from build123d import *

# Parameters (mm, degrees)
SKETCH1_W           = 65
SKETCH1_H           = 32
BOSS_EXTRUDE1_DEPTH = 12
SKETCH10_R          = 3.25
BOLT_EXTRUDE_DEPTH  = 12
SKETCH7_W           = 58
SKETCH7_H           = 27
CUT_EXTRUDE5_DEPTH  = 8
SKETCH8_W           = 5
SKETCH8_H           = 32
BOSS_EXTRUDE3_DEPTH = 11
FILLET6_START       = 3
FILLET6_DEPTH       = 9
FILLET6_START_2     = -16
FILLET6_2_DEPTH     = 4
FILLET6_START_3     = 15
FILLET6_3_DEPTH     = 1
FILLET6_4_ANGLE     = 90
FILLET6_5_ANGLE     = 90
FILLET6_6_ANGLE     = 90
FILLET6_7_ANGLE     = 90
FILLET9_R           = 1
SKETCH11_W          = 120
SKETCH11_H          = 6.033066078
BOSS_EXTRUDE4_DEPTH = 10
SKETCH12_R          = 3.25
BOSS_EXTRUDE5_DEPTH = 12
FILLET11_R          = 7
FILLET12_R          = 3
FILLET13_R          = 3
FILLET15_R          = 1
FILLET16_R          = 1


with BuildPart() as part:
    # Sketch1 → Boss-Extrude1 (new body)
    with BuildSketch(Plane(origin=(0, 0, 0), x_dir=(1, 0, 0), z_dir=(0, 1, 0))):
        with Locations((-32.5, 0)):
            Rectangle(SKETCH1_W, SKETCH1_H)
    extrude(amount=BOSS_EXTRUDE1_DEPTH)

    # Sketch10 → bolt extrude (add)
    with BuildSketch(Plane(origin=(0, 12, 0), x_dir=(1, 0, 0), z_dir=(0, 1, 0))):
        with BuildLine():
            Line((-65, 16), (-70, 16))
            ThreePointArc((-70, 16), (-76.652203093, 14.551570156), (-82.1, 10.468524251))
            Line((-82.1, 10.468524251), (-82.1, -10.468524251))
            ThreePointArc((-82.1, -10.468524251), (-76.652203093, -14.551570156), (-70, -16))
            Line((-70, -16), (-65, -16))
            Line((-65, -16), (-65, 16))
        make_face()
        with Locations(Location((-70.1, -1, 0), (0, 0, 270))):
            Circle(SKETCH10_R, mode=Mode.SUBTRACT)
    extrude(amount=-BOLT_EXTRUDE_DEPTH)

    # Sketch7 → Cut-Extrude5 (cut)
    with BuildSketch(Plane(origin=(0, 12, 0), x_dir=(1, 0, 0), z_dir=(0, 1, 0))):
        with Locations((-29, -1.5)):
            Rectangle(SKETCH7_W, SKETCH7_H)
    extrude(amount=-CUT_EXTRUDE5_DEPTH, mode=Mode.SUBTRACT)

    # Mirror1: part across plane


with BuildPart() as part_1:
    add(part.part)
    add(part.part.mirror(Plane(origin=(0, 0, 0), x_dir=(0, 0, 1), z_dir=(1, 0, 0))))

    # Sketch8 → Boss-Extrude3 (add)
    with BuildSketch(Plane(origin=(0, 4, 0), x_dir=(1, 0, 0), z_dir=(0, 1, 0))):
        Rectangle(SKETCH8_W, SKETCH8_H)
    extrude(amount=BOSS_EXTRUDE3_DEPTH)

    # Fillet6: read off the stored shape, not the designer's step
    # Fillet6 outline → Fillet6 (add)
    with BuildSketch(Plane(origin=(0, 0, 0), x_dir=(1, 0, 0), z_dir=(0, 1, 0)).offset(FILLET6_START)):
        with BuildLine():
            Line((-2.5, -15), (-2.5, -14))
            ThreePointArc((-2.5, -14), (-2.792893219, -14.707106781), (-3.5, -15))
            Line((-3.5, -15), (-2.5, -15))
        make_face()
        with BuildLine():
            ThreePointArc((-3.5, 12), (-2.792893219, 11.707106781), (-2.5, 11))
            Line((-2.5, 11), (-2.5, 12))
            Line((-2.5, 12), (-3.5, 12))
        make_face()
        with BuildLine():
            Line((-58, -15), (-57, -15))
            ThreePointArc((-57, -15), (-57.707106781, -14.707106781), (-58, -14))
            Line((-58, -14), (-58, -15))
        make_face()
        with BuildLine():
            ThreePointArc((-58, 11), (-57.707106781, 11.707106781), (-57, 12))
            Line((-57, 12), (-58, 12))
            Line((-58, 12), (-58, 11))
        make_face()
        with BuildLine():
            Line((2.5, -14), (2.5, -15))
            Line((2.5, -15), (3.5, -15))
            ThreePointArc((3.5, -15), (2.792893219, -14.707106781), (2.5, -14))
        make_face()
        with BuildLine():
            Line((3.5, 12), (2.5, 12))
            Line((2.5, 12), (2.5, 11))
            ThreePointArc((2.5, 11), (2.792893219, 11.707106781), (3.5, 12))
        make_face()
        with BuildLine():
            ThreePointArc((58, -14), (57.707106781, -14.707106781), (57, -15))
            Line((57, -15), (58, -15))
            Line((58, -15), (58, -14))
        make_face()
        with BuildLine():
            Line((58, 12), (57, 12))
            ThreePointArc((57, 12), (57.707106781, 11.707106781), (58, 11))
            Line((58, 11), (58, 12))
        make_face()
    extrude(amount=FILLET6_DEPTH)

    # Fillet6 2 outline → Fillet6 2 (add)
    with BuildSketch(Plane.XY.offset(FILLET6_START_2)):
        with BuildLine():
            Line((-2.5, 12), (-2.5, 13))
            ThreePointArc((-2.5, 13), (-2.792893219, 12.292893219), (-3.5, 12))
            Line((-3.5, 12), (-2.5, 12))
        make_face()
        with BuildLine():
            ThreePointArc((3.5, 12), (2.792893219, 12.292893219), (2.5, 13))
            Line((2.5, 13), (2.5, 12))
            Line((2.5, 12), (3.5, 12))
        make_face()
    extrude(amount=FILLET6_2_DEPTH)

    # Fillet6 3 outline → Fillet6 3 (add)
    with BuildSketch(Plane.XY.offset(FILLET6_START_3)):
        with BuildLine():
            Line((-2.5, 12), (-2.5, 13))
            ThreePointArc((-2.5, 13), (-2.792893219, 12.292893219), (-3.5, 12))
            Line((-3.5, 12), (-2.5, 12))
        make_face()
        with BuildLine():
            ThreePointArc((3.5, 12), (2.792893219, 12.292893219), (2.5, 13))
            Line((2.5, 13), (2.5, 12))
            Line((2.5, 12), (3.5, 12))
        make_face()
    extrude(amount=FILLET6_3_DEPTH)

    # Fillet6 4 outline → Fillet6 4 (revolve)
    with BuildSketch(Plane(origin=(0, 12, 15), x_dir=(0, 0, -1), z_dir=(0, -1, 0))):
        with BuildLine():
            ThreePointArc((0, -3.5), (0.292893219, -2.792893219), (1, -2.5))
            Line((1, -2.5), (0, -2.5))
            Line((0, -2.5), (0, -3.5))
        make_face()
    revolve(axis=Axis((0, 12, 15), (1, 0, 0)), revolution_arc=FILLET6_4_ANGLE)

    # Fillet6 5 outline → Fillet6 5 (revolve)
    with BuildSketch(Plane(origin=(0, 12, -12), x_dir=(0, 1, 0), z_dir=(0, 0, -1))):
        with BuildLine():
            ThreePointArc((0, -3.5), (0.292893219, -2.792893219), (1, -2.5))
            Line((1, -2.5), (0, -2.5))
            Line((0, -2.5), (0, -3.5))
        make_face()
    revolve(axis=Axis((0, 12, -12), (1, 0, 0)), revolution_arc=FILLET6_5_ANGLE)

    # Fillet6 6 outline → Fillet6 6 (revolve)
    with BuildSketch(Plane(origin=(0, 12, -12), x_dir=(0, 1, 0), z_dir=(0, 0, -1))):
        with BuildLine():
            Line((0, 2.5), (1, 2.5))
            ThreePointArc((1, 2.5), (0.292893219, 2.792893219), (0, 3.5))
            Line((0, 3.5), (0, 2.5))
        make_face()
    revolve(axis=Axis((0, 12, -12), (1, 0, 0)), revolution_arc=FILLET6_6_ANGLE)

    # Fillet6 7 outline → Fillet6 7 (revolve)
    with BuildSketch(Plane(origin=(0, 12, 15), x_dir=(0, 0, -1), z_dir=(0, -1, 0))):
        with BuildLine():
            Line((0, 2.5), (1, 2.5))
            ThreePointArc((1, 2.5), (0.292893219, 2.792893219), (0, 3.5))
            Line((0, 3.5), (0, 2.5))
        make_face()
    revolve(axis=Axis((0, 12, 15), (1, 0, 0)), revolution_arc=FILLET6_7_ANGLE)

    # Fillet9
    fillet9_edges = [part_1.edges().sort_by_distance(p)[0] for p in [
        (2.5, 15, 0),
        (0, 15, -16),
        (-2.5, 15, 0),
        (0, 15, 16),
    ]]
    fillet(fillet9_edges, radius=FILLET9_R)

    # Sketch11 → Boss-Extrude4 (add)
    with BuildSketch(Plane.XZ):
        Polygon((70.002161454, 12.077158354), (-70.005398194, 12), (-70, 16), (70, 16), align=None)
        Rectangle(SKETCH11_W, SKETCH11_H)
        Polygon((70.002161454, -12.077158354), (70, -16), (-70, -16), (-70.005398194, -12), align=None)
    extrude(amount=BOSS_EXTRUDE4_DEPTH)

    # Sketch12 → Boss-Extrude5 (add)
    with BuildSketch(Plane.XZ):
        with BuildLine():
            Line((-8, -12), (-8, -22))
            ThreePointArc((-8, -22), (0, -30), (8, -22))
            Line((8, -22), (8, -12))
            Line((8, -12), (-8, -12))
        make_face()
        with Locations(Location((0, -22, 0), (0, 0, 270))):
            Circle(SKETCH12_R, mode=Mode.SUBTRACT)
    extrude(amount=-BOSS_EXTRUDE5_DEPTH)

    # Fillet11
    fillet11_edges = [part_1.edges().sort_by_distance(p)[0] for p in [
        (-70.002699097, 0, -14),
        (70.001080727, 0, -14.038579177),
        (-70.002699097, 0, 14),
        (70.001080727, 0, 14.038579177),
    ]]
    fillet(fillet11_edges, radius=FILLET11_R)

    # Fillet12
    fillet12_edges = [part_1.edges().sort_by_distance(p)[0] for p in [
        (0, 0, 3.016533039),
        (0, 0, -3.016533039),
        (-0.001624692, 0, 12.038579173),
        (-0.001624692, 0, -12.038579173),
    ]]
    fillet(fillet12_edges, radius=FILLET12_R)

    # Fillet13
    fillet13_edges = [part_1.edges().sort_by_distance(p)[0] for p in [
        (-8, 6, -16),
        (8, 6, -16),
    ]]
    fillet(fillet13_edges, radius=FILLET13_R)

    # Fillet15
    fillet15_edges = [part_1.edges().sort_by_distance(p)[0] for p in [
        (0, 0, -16),
    ]]
    fillet(fillet15_edges, radius=FILLET15_R)

    # Fillet16
    fillet16_edges = [part_1.edges().sort_by_distance(p)[0] for p in [
        (60, 0, 0),
        (-60, 0, 0),
    ]]
    fillet(fillet16_edges, radius=FILLET16_R)


solid = part_1.part
The model under review builds one solid part; all positions refer to its coordinate system, in mm. A direction names the side the tool comes from. Coordinates: 2 decimals unless noted, no trailing zeros. Loops run counter-clockwise (first coordinate to the right, second up) from the corner with the lowest first, then second, coordinate; pieces in that order, holes last.
(1) Consider section B-B, the plane z = -7.5. Give the boundary of the cut face in (x, y), plus the area to 3 significant figures.
Determined:
outline: (-82.1, 0) - (82.1, 0) - (82.1, 12) - (58, 12) - (58, 4) - (2.5, 4) - (2.5, 14) arc R1 ccw to (1.5, 15) - (-1.5, 15) arc R1 ccw to (-2.5, 14) - (-2.5, 4) - (-58, 4) - (-58, 12) - (-82.1, 12) - close
area: 1,100 mm2
(2) Wall thickness on L1, parallel to Z at x = -12.5, y = -8.25: over which ranges is the line inside the solid? List them lowest first.
Determined:
L1: z = -16 to -12.03, -3.02 to 3.02, 12.03 to 16
(3) Insertion check: P1, Ø2.5, axis at x = 21.5, y = 8, coming from the -Z side; P2, Ø3.5, axis at y = 8.5, z = -20.5, coming from the +X side; P3, Ø1.5, axis at x = -22.5, z = -10, coming from the +Y side; P4, Ø5, axis at x = 0, z = -22, coming from the +Y side. Each pin has a flat end and moves straight along its axis. Give the tip position at first contact, or say it passes through.
Determined:
P1: stops at z = -16
P2: stops at x = 8.01
P3: stops at y = 4
P4: passes through
(4) Tool access review of faces 1 (the cylindrical face through (0.854, -0.855, 3.919)), 2 (the flat face through (0.4, 0, -6.5)), 3 (the flat face through (-60, -5, 0)), 4 (the flat face through (-30, 8, 15)): name each direction out of +Z, -Z, +X, -X, +Y, -Y from which nothing blocks a thin tool from reaching the whole face with its end or side.
Determined:
face 1: +X, -X, -Y
face 2: -Y
face 3: -X, -Y
face 4: +Y
(5) Draft analysis for pull direction X (two halves, no side actions). For faces 5 (the cylindrical face through (8.86, 5.41, -16.9)), 6 (the flat face through (-1, -6, 3.017)), 7 (the cylindrical face through (-66.878, 6.084, 0.577)), state which applies: +X half, -X half, draft (parallel to the pull), parting line (faces both ways), or undercut.
Determined:
face 5: +X half
face 6: draft
face 7: undercut
(6) Consider section A-A, the plane z = 1. Give the boundary of the cut face in (x, y).
Determined:
outline: (-82.1, 0) - (-73.35, 0) - (-73.35, 12) - (-82.1, 12) - close; (-66.85, 0) - (-61, 0) arc R1 cw to (-60, -1) - (-60, -10) - (60, -10) - (60, -1) arc R1 cw to (61, 0) - (66.85, 0) - (66.85, 12) - (58, 12) - (58, 4) - (2.5, 4) - (2.5, 14) arc R1 ccw to (1.5, 15) - (-1.5, 15) arc R1 ccw to (-2.5, 14) - (-2.5, 4) - (-58, 4) - (-58, 12) - (-66.85, 12) - close; (73.35, 0) - (82.1, 0) - (82.1, 12) - (73.35, 12) - close
